The model under review builds one solid part; all positions refer to its coordinate system, in mm. A direction names the side the tool comes from. Round coordinates to 2 decimals unless told otherwise and drop trailing zeros. Loops run counter-clockwise (first coordinate to the right, second up) from the corner with the lowest first, then second, coordinate; pieces in that order, holes last. Notation, with made-up numbers: M 23,-8.75 L 35,-8.75 A17 ccw 35,2.25 Z; hole C 0,-21 d8. An arc over 180 degrees is marked long. Return JSON: item names as keys, results as strings. Group by question number.
Q1. Clearance check with flat-ended pins moving along their axes: pin 1 Ø0.7 at (y, z) = (16.5, 1) entering from -X; pin 2 Ø3 at (x, y) = (10, -8.5) entering from +Z; pin 3 Ø0.7 at (y, z) = (15, 1.5) entering from +X. State where each tip first meets the part, or that it passes through.
Q2. For faces 5 (the face through (5.25, 18, 1)), 6 (the face through (-5.25, 18, 1)), 7 (the face through (0, 0, -5)), list the 3-axis set-ups (+Z, -Z, +X, -X, +Y, -Y) from which the entire face can be reached by the end or side of a thin tool; tool diameter is ignored.
Q3. Consider section D-D (y = 12.5). State the section outline as (x, z) points.
Q4. To check wall thickness, follow line 1 along Y through (x, z) = (-25, -2.4); line 2 along Y through (x, z) = (-9, -3.1). State the ranges of each line that lie inside material, in increasing order.
Q5. Consider section A-A (z = -2.75). Count the separate pieces of the cut face and the enclosed holes in it, and give its area (3 significant figures).
Q6. Draft analysis for pull direction Y (two halves, no side actions). For faces 1 (the face through (0, -30, -2)), 2 (the face through (0, 5.5, 1)), 3 (the face through (0, 18, 2.25)), 4 (the face through (0, -5.5, 1)), state which applies: pulls with the +Y half, pulls with the -Y half, needs draft (parallel to the pull), parting line crosses it, or undercut.
Q7. Consider section C-C (x = -2). State the section outline as (y, z) points, and give its area (3 significant figures).
Q8. Consider section B-B (y = 26.5). State the section outline as (x, z) points, and give its area (3 significant figures).
from build123d import *

# Parameters (mm, degrees)
F1_DEPTH = 5
F2_W     = 10.5
F2_H     = 24.5
F3_DEPTH = 2.25


# Not quite as in the source:
# - a feature names something its author has since deleted; it is built from what else it names


with BuildPart() as f1:
    # F0 (on Top) → F1 (new body)
    with BuildSketch(Plane.XY):
        Polygon((5.25, -30), (30, -30), (30, 30), (-30, 30), (-30, -30), (0, -30), align=None)
        with BuildLine():
            Line((22.5, -25), (-22.5, -25))
            ThreePointArc((-22.5, -25), (-26.767766953, -26.767766953), (-25, -22.5))
            Line((-25, -22.5), (-25, 22.5))
            ThreePointArc((-25, 22.5), (-26.767766953, 26.767766953), (-22.5, 25))
            Line((-22.5, 25), (22.5, 25))
            ThreePointArc((22.5, 25), (25, 27.5), (27.5, 25))
            ThreePointArc((27.5, 25), (26.767766953, 23.232233047), (25, 22.5))
            Line((25, 22.5), (25, -22.5))
            ThreePointArc((25, -22.5), (26.767766953, -23.232233047), (27.5, -25))
            ThreePointArc((27.5, -25), (25, -27.5), (22.5, -25))
        make_face(mode=Mode.SUBTRACT)
        with BuildLine():
            ThreePointArc((-25, -22.5), (-23.232233047, -23.232233047), (-22.5, -25))
            Line((-22.5, -25), (22.5, -25))
            ThreePointArc((22.5, -25), (23.232233047, -23.232233047), (25, -22.5))
            Line((25, -22.5), (25, 22.5))
            ThreePointArc((25, 22.5), (23.232233047, 23.232233047), (22.5, 25))
            Line((22.5, 25), (-22.5, 25))
            ThreePointArc((-22.5, 25), (-23.232233047, 23.232233047), (-25, 22.5))
            Line((-25, 22.5), (-25, -22.5))
        make_face()
        with BuildLine():
            Line((6.5, -9), (-6.5, -9))
            ThreePointArc((-6.5, -9), (-10.767766953, -10.767766953), (-9, -6.5))
            Line((-9, -6.5), (-9, 6.5))
            ThreePointArc((-9, 6.5), (-10.767766953, 10.767766953), (-6.5, 9))
            Line((-6.5, 9), (6.5, 9))
            ThreePointArc((6.5, 9), (9, 11.5), (11.5, 9))
            ThreePointArc((11.5, 9), (10.767766953, 7.232233047), (9, 6.5))
            Line((9, 6.5), (9, -6.5))
            ThreePointArc((9, -6.5), (10.767766953, -7.232233047), (11.5, -9))
            ThreePointArc((11.5, -9), (9, -11.5), (6.5, -9))
        make_face(mode=Mode.SUBTRACT)
        with BuildLine():
            ThreePointArc((-9, -6.5), (-7.232233047, -7.232233047), (-6.5, -9))
            Line((-6.5, -9), (6.5, -9))
            ThreePointArc((6.5, -9), (7.232233047, -7.232233047), (9, -6.5))
            Line((9, -6.5), (9, 6.5))
            ThreePointArc((9, 6.5), (7.232233047, 7.232233047), (6.5, 9))
            Line((6.5, 9), (-6.5, 9))
            ThreePointArc((-6.5, 9), (-7.232233047, 7.232233047), (-9, 6.5))
            Line((-9, 6.5), (-9, -6.5))
        make_face()
    extrude(amount=-F1_DEPTH)

    # F2 (on face) → F3 (join)
    with BuildSketch(Plane.XY):
        with Locations((0, 17.75)):
            Rectangle(F2_W, F2_H)
        with Locations((0, -17.75)):
            Rectangle(F2_W, F2_H)
    extrude(amount=F3_DEPTH)


solid = f1.part
Values:
{
 "1": {"pin 1": "stops at x = -5.25", "pin 2": "stops at z = 0", "pin 3": "stops at x = 5.25"},
 "2": {"face 5": "+Z, +X, +Y, -Y", "face 6": "+Z, -X, +Y, -Y", "face 7": "-Z, +X, -X, +Y, -Y"},
 "3": {"outline": "M -30,-5 L 30,-5 L 30,0 L 5.25,0 L 5.25,2.25 L -5.25,2.25 L -5.25,0 L -30,0 Z"},
 "4": {"line 1": "y = -30 to -27.5, -22.5 to 22.5, 27.5 to 30", "line 2": "y = -30 to -11.5, -6.5 to 6.5, 11.5 to 30"},
 "5": {"separate pieces": "1", "enclosed holes": "8", "area": "3,440 mm2"},
 "6": {"face 1": "pulls with the -Y half", "face 2": "undercut", "face 3": "needs draft", "face 4": "undercut"},
 "7": {"outline": "M -30,-5 L 30,-5 L 30,2.25 L 5.5,2.25 L 5.5,0 L -5.5,0 L -5.5,2.25 L -30,2.25 Z", "area": "410 mm2"},
 "8": {"outline": "M -30,-5 L -27,-5 L -27,0 L -30,0 Z; M -23,-5 L 23,-5 L 23,0 L 5.25,0 L 5.25,2.25 L -5.25,2.25 L -5.25,0 L -23,0 Z; M 27,-5 L 30,-5 L 30,0 L 27,0 Z", "area": "284 mm2"}
}
